```python
from build123d import *

# Parameters (mm, degrees)
SKETCH1_W           = 40
SKETCH1_H           = 100
BOSS_EXTRUDE1_DEPTH = 10
SKETCH3_R           = 2.5
CUT_EXTRUDE1_DEPTH  = 40
SKETCH4_R           = 5
CUT_EXTRUDE2_DEPTH  = 6
SKETCH6_R           = 5
CUT_EXTRUDE3_DEPTH  = 6
SKETCH7_R           = 3
CUT_EXTRUDE4_DEPTH  = 5


with BuildPart() as part:
    # Sketch1 → Boss-Extrude1 (new body)
    with BuildSketch(Plane.XY):
        with Locations((20, 50)):
            Rectangle(SKETCH1_W, SKETCH1_H)
    extrude(amount=BOSS_EXTRUDE1_DEPTH)

    # Sketch3 → Cut-Extrude1 (cut)
    with BuildSketch(Plane.XY.offset(10)):
        with Locations((8.3, 61.7)):
            Circle(SKETCH3_R)
        with Locations((31.7, 61.7)):
            Circle(SKETCH3_R)
        with Locations((31.7, 38.3)):
            Circle(SKETCH3_R)
        with Locations((8.3, 38.3)):
            Circle(SKETCH3_R)
    extrude(amount=-CUT_EXTRUDE1_DEPTH, mode=Mode.SUBTRACT)

    # Sketch4 → Cut-Extrude2 (cut)
    with BuildSketch(Plane.XY.offset(10)):
        with Locations((8.3, 61.7)):
            Circle(SKETCH4_R)
        with Locations((31.7, 61.7)):
            Circle(SKETCH4_R)
        with Locations((31.7, 38.3)):
            Circle(SKETCH4_R)
        with Locations((8.3, 38.3)):
            Circle(SKETCH4_R)
    extrude(amount=-CUT_EXTRUDE2_DEPTH, mode=Mode.SUBTRACT)

    # Sketch6 → Cut-Extrude3 (cut)
    with BuildSketch(Plane(origin=(0, 0, 0), x_dir=(-1, 0, 0), z_dir=(0, 0, -1))):
        with Locations((-20, 85)):
            Circle(SKETCH6_R)
        with Locations((-20, 15)):
            Circle(SKETCH6_R)
    extrude(amount=-CUT_EXTRUDE3_DEPTH, mode=Mode.SUBTRACT)

    # Sketch7 → Cut-Extrude4 (cut, through all)
    with BuildSketch(Plane(origin=(0, 0, 6), x_dir=(-1, 0, 0), z_dir=(0, 0, -1))):
        with Locations((-20, 15)):
            Circle(SKETCH7_R)
        with Locations((-20, 85)):
            Circle(SKETCH7_R)
    extrude(amount=-CUT_EXTRUDE4_DEPTH, mode=Mode.SUBTRACT)


solid = part.part
```
Check sheet for the modelled part. Datum: model origin and axes. Units: mm. A direction names the side the tool comes from. Round coordinates to 2 decimals unless told otherwise and drop trailing zeros. Order: outer loops, then holes, each group sorted by start corner. A loop starts at its lowest first (then second) coordinate and runs counter-clockwise, first axis right, second up.
1) Scan lines: line 1 (Y direction, x = 20, z = 2.3); line 2 (Y direction, x = 8.3, z = 6.1); line 3 (X direction, y = 89, z = 5). Record each from-to range of solid material in increasing order.
2) Section check C-C (y = 38.3). Record the boundary of the cut face in (x, z), and give its area (3 significant figures).
3) Tool access check on faces 5 (the flat face through (20, 51, 0)), 6 (the cylindrical face through (27.7, 58.7, 7)), 7 (the cylindrical face through (21.08, 10.12, 2.96)). Record the directions out of +Z, -Z, +X, -X, +Y, -Y that give a thin tool (end or side, any length) a straight path to the whole face; none if there is none.
4) Section check D-D (y = 15). Record the boundary of the cut face in (x, z).
5) Section check A-A (x = 20). Record the boundary of the cut face in (y, z), and give its area (3 significant figures).
6) Mould release check, pull along X, two halves, no side actions. Record for faces 1 (the flat face through (20.1, 11.7, 6)), 2 (the flat face through (40, 49, 5)), 3 (the flat face through (20, 51, 10)), 4 (the flat face through (0, 49, 5)): +X half, -X half, draft (parallel to the pull), parting line (faces both ways), or undercut.
7) Section check B-B (z = 7). Record the boundary of the cut face in (x, y).
8) Go/stop test with flat-tipped pins: pin 1 Ø8 at (x, y) = (20, 85) entering from -Z; pin 2 Ø5 at (x, y) = (32, 40) entering from +Z; pin 3 Ø11.5 at (x, y) = (20, 85) entering from -Z. Record where each tip stops, or that it passes through.
Result:
1. line 1: y = 0 to 10, 20 to 80, 90 to 100
1. line 2: y = 0 to 33.3, 43.3 to 56.7, 66.7 to 100
1. line 3: x = 0 to 17, 23 to 40
2. outline: (0, 0) - (5.8, 0) - (5.8, 4) - (3.3, 4) - (3.3, 10) - (0, 10) - close; (10.8, 0) - (29.2, 0) - (29.2, 4) - (26.7, 4) - (26.7, 10) - (13.3, 10) - (13.3, 4) - (10.8, 4) - close; (34.2, 0) - (40, 0) - (40, 10) - (36.7, 10) - (36.7, 4) - (34.2, 4) - close
2. area: 240 mm2
3. face 5: -Z, +X, -X, +Y, -Y
3. face 6: +Z
3. face 7: -Z
4. outline: (0, 0) - (15, 0) - (15, 6) - (17, 6) - (17, 10) - (0, 10) - close; (23, 6) - (25, 6) - (25, 0) - (40, 0) - (40, 10) - (23, 10) - close
5. outline: (0, 0) - (10, 0) - (10, 6) - (12, 6) - (12, 10) - (0, 10) - close; (18, 6) - (20, 6) - (20, 0) - (80, 0) - (80, 6) - (82, 6) - (82, 10) - (18, 10) - close; (88, 6) - (90, 6) - (90, 0) - (100, 0) - (100, 10) - (88, 10) - close
5. area: 832 mm2
6. face 1: undercut
6. face 2: +X half
6. face 3: draft
6. face 4: -X half
7. outline: (0, 0) - (40, 0) - (40, 100) - (0, 100) - close; hole circle Ø10 at (8.3, 38.3); hole circle Ø10 at (8.3, 61.7); hole circle Ø6 at (20, 15); hole circle Ø6 at (20, 85); hole circle Ø10 at (31.7, 38.3); hole circle Ø10 at (31.7, 61.7)
8. pin 1: stops at z = 6
8. pin 2: stops at z = 4
8. pin 3: stops at z = 0
